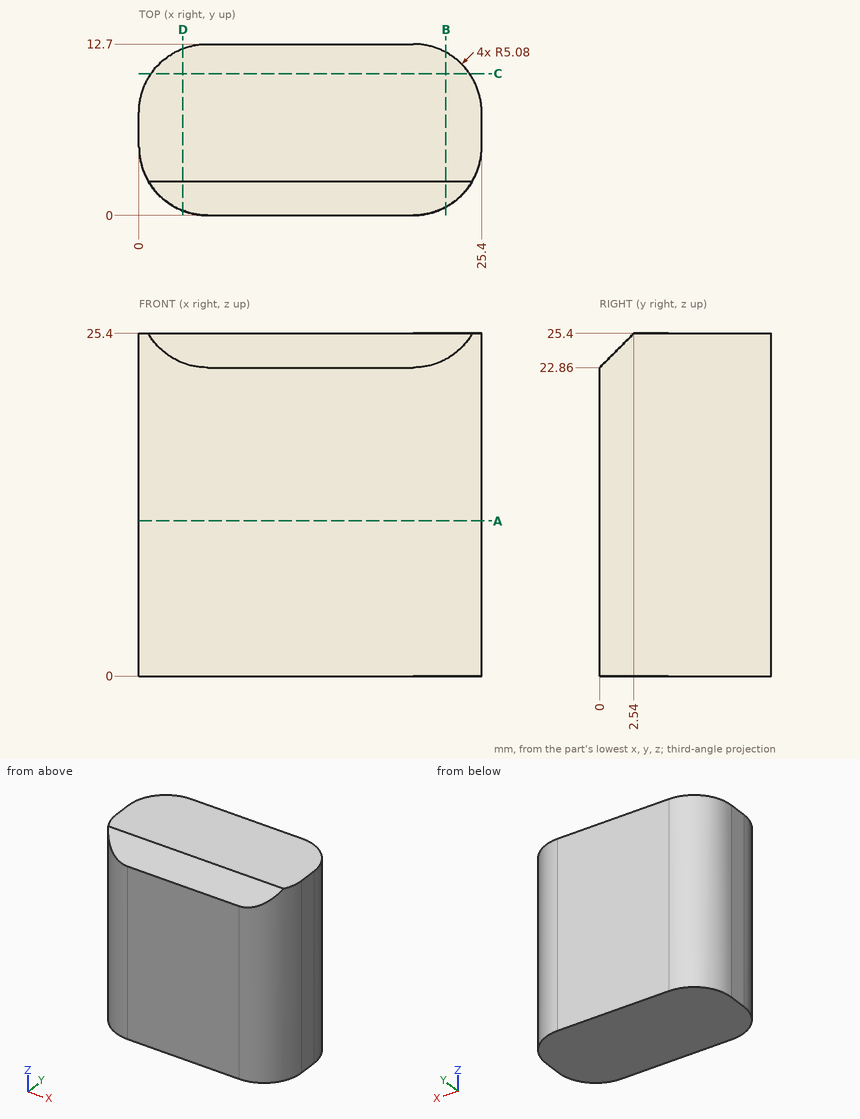
Answer from the drawing. Dimensions are ordinates in mm from the lowest x, y and z of the part. Give positions to 0.01 mm unless a question says otherwise; leave off trailing zeros. Order: outer loops, then holes, each group sorted by start corner. A loop starts at its lowest first (then second) coordinate and runs counter-clockwise, first axis right, second up. Notation, with made-up numbers: (49.25, -27.5) -> (89.25, -27.5) arc R23 ccw to (89.25, -14.5) -> close; hole circle Ø3 at (34.5, 2.25). An arc over 180 degrees is marked (long way). Answer as a JSON object with one key per item and string values. Group by question number.
1. Flat-ended cylindrical pins translate along their axes: pin 1 Ø4 at (x, y) = (7, 4.5) entering from -Z; pin 2 Ø1 at (y, z) = (9.5, 17) entering from -X; pin 3 Ø5 at (x, z) = (23, 21.5) entering from -Y. Find the tip coordinate at first contact, or state that the pin passes through.
2. Consider line 1 along Y through (x, z) = (5, 21); line 2 along X through (y, z) = (11.25, 1); line 3 along X through (y, z) = (11, 21.5). Determine where each line is inside the solid, lowest interval first. Write a range as [from, to].
3. Section A-A on z = 11.5 is taken. Determine the outline of the cut face in (x, y), plus the area to 3 significant figures.
4. Section D-D on x = 3.25 is taken. Determine the outline of the cut face in (y, z), plus the area to 3 significant figures.
5. Section C-C on y = 10.5 is taken. Determine the outline of the cut face in (x, z).
6. Section B-B on x = 22.75 is taken. Determine the outline of the cut face in (y, z).
Result sheet:
{
 "1": {"pin 1": "stops at z = 0", "pin 2": "stops at x = 0.19", "pin 3": "stops at y = 0"},
 "2": {"line 1": "y = [0, 12.7]", "line 2": "x = [1.53, 23.87]", "line 3": "x = [1.29, 24.11]"},
 "3": {"outline": "(0, 5.08) arc R5.08 ccw to (5.08, 0) -> (20.32, 0) arc R5.08 ccw to (25.4, 5.08) -> (25.4, 7.62) arc R5.08 ccw to (20.32, 12.7) -> (5.08, 12.7) arc R5.08 ccw to (0, 7.62) -> close", "area": "300 mm^2"},
 "4": {"outline": "(0.34, 0) -> (12.36, 0) -> (12.36, 25.4) -> (2.54, 25.4) -> (0.34, 23.2) -> close", "area": "303 mm^2"},
 "5": {"outline": "(0.9, 0) -> (24.5, 0) -> (24.5, 25.4) -> (0.9, 25.4) -> close"},
 "6": {"outline": "(0.62, 0) -> (12.08, 0) -> (12.08, 25.4) -> (2.54, 25.4) -> (0.62, 23.48) -> close"}
}
